CAD build for the part. Positions are in the model's coordinates, mm. Face numbers are marked on the shaded views. Coordinates: 2 decimals unless noted, no trailing zeros. Write each loop counter-clockwise with the first axis right and the second up, starting at its lowest first coordinate (ties: lowest second). Pieces come first, ordered by that corner, then holes. Notation, with made-up numbers: (-1, 67.25) - (21, 67.25) arc R22 cw to (21, 86.25) - close; hole circle Ø7 at (-9, 35.25). An arc over 180 degrees is marked (long way). One line per question, with ' | ' between items. Start each with the question number.
1. Band-saw the part on B-B, the plane z = 10. Give the number of separate pieces and of enclosed holes in the cut face, then the cut area to 3 significant figures.
2. Probe line 1 (X direction, y = 339.5, z = 3); line 2 (Z direction, x = 53.5, y = 352); line 3 (Y direction, x = 149.5, z = 24). List the from-to ranges inside material, lowest first.
3. Two-plate mould, pull along Y, no slides. Class the marked faces 1 and 2: +Y half, -Y half, draft (parallel to the pull), parting line (faces both ways), or undercut.
4. Flat gauge pins, fed straight in: P1, Ø5, axis at y = 352.5, z = 19.5, coming from the -X side; P2, Ø12, axis at x = 155.5, y = 383, coming from the +Z side; P3, Ø1, axis at x = -155, z = 16, coming from the +Y side. Where does each tip first touch, or does it go through?
5. Band-saw the part on A-A, the plane y = 361.5. Write the cut outline in (x, z).
from build123d import *

# Parameters (mm, degrees)
BOSS_EXTRUDE1_DEPTH = 21
SKETCH2_R           = 30
CUT_EXTRUDE1_DEPTH  = 527.362693656
SKETCH4_R           = 40
SKETCH4_R_2         = 30
BOSS_EXTRUDE3_DEPTH = 10


with BuildPart() as part:
    # Sketch1 → Boss-Extrude1 (new body)
    with BuildSketch(Plane.XY):
        with BuildLine():
            ThreePointArc((-267.733324074, 386.480114093), (-317.733324074, 336.480114093), (-267.733324074, 286.480114093))
            add(Edge.make_bspline(
                [(-267.733324074, 286.480114093), (-61.536299878, 365.758634067), (152.142574227, 266.270803333)],
                knots=[0, 0, 0, 1, 1, 1], degree=2))
            ThreePointArc((152.142574227, 266.270803333), (212.142574227, 326.270803333), (152.142574227, 386.270803333))
            add(Edge.make_bspline(
                [(-267.733324074, 386.480114093), (-58.376892778, 451.86591416), (152.142574227, 386.270803333)],
                knots=[0, 0, 0, 1, 1, 1], degree=2))
        make_face()
    extrude(amount=BOSS_EXTRUDE1_DEPTH)

    # Sketch2 → Cut-Extrude1 (cut, through all)
    with BuildSketch(Plane.XY):
        with Locations(Location((-267.733324074, 336.480114093, 0), (0, 0, 180))):
            Circle(SKETCH2_R)
        with Locations(Location((152.142574227, 326.270803333, 0), (0, 0, 180))):
            Circle(SKETCH2_R)
    extrude(amount=CUT_EXTRUDE1_DEPTH, mode=Mode.SUBTRACT)

    # Sketch4 → Boss-Extrude3 (add)
    with BuildSketch(Plane.XY.offset(21)):
        with Locations((152.142574227, 326.270803333)):
            Circle(SKETCH4_R)
        with Locations(Location((152.142574227, 326.270803333, 0), (0, 0, 180))):
            Circle(SKETCH4_R_2, mode=Mode.SUBTRACT)
    extrude(amount=BOSS_EXTRUDE3_DEPTH)


solid = part.part
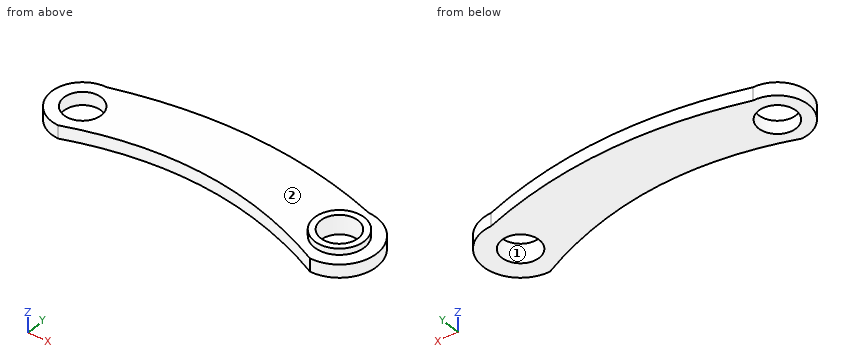
Filled in:
1) separate pieces: 1 | enclosed holes: 2 | area: 46,800 mm²
2) line 1: x = -317.64 to -297.58, -237.89 to 125.22, 179.07 to 210.67 | line 2: z = 0 to 21 | line 3: y = 286.36 to 296.39, 356.15 to 366.18
3) face 1: undercut | face 2: draft
4) P1: stops at x = -315.87 | P2: stops at z = 21 | P3: stops at y = 412.25
5) outline: (-311.02, 0) - (-284.29, 0) - (-284.29, 21) - (-311.02, 21) - close; (-251.18, 0) - (200.71, 0) - (200.71, 21) - (171.09, 21) - (171.09, 31) - (133.2, 31) - (133.2, 21) - (-251.18, 21) - close
